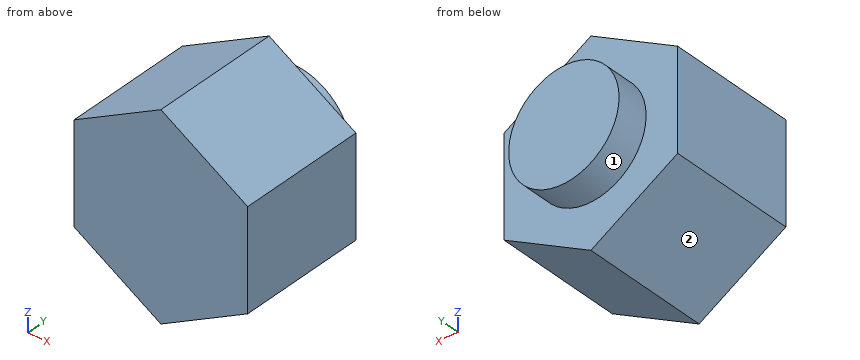
Autodesk Inventor part; units mm, degrees
ref_plane "YZ Plane" through (0, 0, 0) normal (1, 0, 0) x (0, 1, 0)
ref_plane "XZ Plane" through (0, 0, 0) normal (0, 1, 0) x (-1, 0, 0)
ref_plane "XY Plane" through (0, 0, 0) normal (0, 0, 1) x (1, 0, 0)
sketch "Sketch1" plane through (0, 0, 0) normal (0, 1, 0) x (-1, 0, 0)
  line L0 (5.5, -3.1754) -> (0, -6.3509)
  line L1 (0, -6.3509) -> (-5.5, -3.1754)
  line L2 (-5.5, -3.1754) -> (-5.5, 3.1754)
  line L3 (-5.5, 3.1754) -> (0, 6.3509)
  line L4 (0, 6.3509) -> (5.5, 3.1754)
  line L5 (5.5, 3.1754) -> (5.5, -3.1754)
  circle A0 centre (0, 0) radius 3.5
  dimension "d0" = 7
  dimension "d1" = 11
extrude "Extrusion1" add sketch "Sketch1" against normal blind 8 contours L0 L1 L2 L3 L4 L5 | A0
extrude "Extrusion2" add sketch "Sketch1" along normal blind 2 contours A0
properties part number "EccentricNut 5mmID 11mmHex" material "Aluminum 6061"
Read the model definition and answer for the solid it produces. Units are mm, in the model's axes. Face numbers are marked on the shaded views. A direction names the side the tool comes from. Round coordinates to 2 decimals unless told otherwise and drop trailing zeros. Write each loop counter-clockwise with the first axis right and the second up, starting at its lowest first coordinate (ties: lowest second). Pieces come first, ordered by that corner, then holes. Notation, with made-up numbers: M 55.25,-14.75 L 73.25,-14.75 A3 ccw 73.25,-10.75 Z; hole C 18.25,34.25 d11. An arc over 180 degrees is marked long. One line per item, written item: value.
Q1. Find section B-B on z = 0. Write down the section's boundary in (x, y).
Data:
outline: M -5.5,-8 L 5.5,-8 L 5.5,0 L 3.5,0 L 3.5,2 L -3.5,2 L -3.5,0 L -5.5,0 Z
Q2. Flat-ended cylindrical pins translate along their axes: pin 1 Ø6 at (x, y) = (-3.5, -4.5) entering from -Z; pin 2 Ø1.5 at (x, z) = (2.5, 4) entering from +Y; pin 3 Ø6 at (x, y) = (-4, -0.5) entering from +Z. Find the tip coordinate at first contact, or state that the pin passes through.
Data:
pin 1: z = -6.06
pin 2: y = 0
pin 3: z = 5.77
Q3. Find section D-D on z = -5.5. Write down the section's boundary in (x, y), plus the area to 3 significant figures.
Data:
outline: M -1.47,-8 L 1.47,-8 L 1.47,0 L -1.47,0 Z
area: 23.6 mm2
Q4. Straight lines are drawn through the part: line 1 (Y direction, x = -3.75, z = 1.75); line 2 (Z direction, x = -0.5, y = -6.75); line 3 (Z direction, x = 2, y = -2). For each, find the intervals that lie inside material, in ascending order. Write a range as [from, to].
Data:
line 1: [-8, 0]
line 2: [-6.06, 6.06]
line 3: [-5.2, 5.2]
Q5. Find section A-A on y = -3.75. Write down the section's boundary in (x, z).
Data:
outline: M -5.5,-3.18 L 0,-6.35 L 5.5,-3.18 L 5.5,3.18 L 0,6.35 L -5.5,3.18 Z
Q6. Find section C-C on x = 3.25. Write down the section's boundary in (y, z), plus the area to 3 significant figures.
Data:
outline: M -8,-4.47 L 0,-4.47 L 0,-1.3 L 2,-1.3 L 2,1.3 L 0,1.3 L 0,4.47 L -8,4.47 Z
area: 76.8 mm2
Q7. Which of the six approach directions +Z, -Z, +X, -X, +Y, -Y give full straight-line access (tool end or side, diameter ignored) to the marked faces 1 and 2?
Data:
face 1: +Y
face 2: -Z, -X, +Y, -Y
